from build123d import *

# Parameters (mm, degrees)
PAD_DEPTH          = 11
SKETCH001_R        = 2
PAD001_DEPTH       = 0.4
SKETCH002_R        = 0.5
PAD002_DEPTH       = 3.8
SKETCH003_R        = 0.5
POCKET_DEPTH       = 3
SKETCH004_R        = 2.5
SKETCH004_R_2      = 1
PAD003_DEPTH       = 1.2
SKETCH005_W        = 3
SKETCH005_H        = 1.8
POCKET001_DEPTH    = 2
SKETCH006_W        = 0.3
SKETCH006_H        = 1.478048
PAD004_DEPTH       = 2
POCKET002_DEPTH    = 0.2
POLARPATTERN_COUNT = 2


with BuildPart() as part:
    # Sketch → Pad (new body, symmetric)
    with BuildSketch(Plane.XY):
        with BuildLine():
            ThreePointArc((-3.316625, 5), (-6, 0), (-3.316625, -5))
            Line((-3.316625, -5), (3.316625, -5))
            ThreePointArc((3.316625, -5), (6, 0), (3.316625, 5))
            Line((-3.316625, 5), (3.316625, 5))
        make_face()
    extrude(amount=PAD_DEPTH, both=True)

    # Sketch001 (on Face6 of Pad) → Pad001 (join)
    with BuildSketch(Plane.XY.offset(11)):
        Circle(SKETCH001_R)
    extrude(amount=PAD001_DEPTH)

    # Sketch002 (on Face8 of Pad001) → Pad002 (join)
    with BuildSketch(Plane.XY.offset(11.4)):
        Circle(SKETCH002_R)
    extrude(amount=PAD002_DEPTH)

    # Sketch003 (on Face5 of Pad002) → Pocket (cut)
    with BuildSketch(Plane.XY.offset(11)):
        with Locations((0, 3.6)):
            Circle(SKETCH003_R)
        with Locations((-4.3, 0)):
            Circle(SKETCH003_R)
        with Locations((4.3, 0)):
            Circle(SKETCH003_R)
    extrude(amount=-POCKET_DEPTH, mode=Mode.SUBTRACT)

    # Sketch004 (on Face4 of Pocket) → Pad003 (join)
    with BuildSketch(Plane(origin=(0, 0, -11), x_dir=(1, 0, 0), z_dir=(0, 0, -1))):
        Circle(SKETCH004_R)
        Circle(SKETCH004_R_2, mode=Mode.SUBTRACT)
    extrude(amount=PAD003_DEPTH)

    # Sketch005 (on Face4 of Pad003) → Pocket001 (cut)
    with BuildSketch(Plane(origin=(0, 0, -11), x_dir=(1, 0, 0), z_dir=(0, 0, -1))):
        with Locations((-6, 0)):
            Rectangle(SKETCH005_W, SKETCH005_H)
        with Locations((6, 0)):
            Rectangle(SKETCH005_W, SKETCH005_H)
    extrude(amount=-POCKET001_DEPTH, mode=Mode.SUBTRACT)

    # Sketch006 (on Face2 of Pocket001) → Pad004 (join)
    with BuildSketch(Plane(origin=(0, 0, -11), x_dir=(1, 0, 0), z_dir=(0, 0, -1))):
        with Locations((-3.95, 0)):
            Rectangle(SKETCH006_W, SKETCH006_H)
        with Locations((3.95, 0)):
            Rectangle(SKETCH006_W, SKETCH006_H)
    extrude(amount=PAD004_DEPTH)

    # Sketch007 (on Face6 of Pad004) → Pocket002 (cut)
    with BuildSketch(Plane.XZ.offset(5)):
        with BuildLine():
            ThreePointArc((-2.15, 2.4), (-2.4, 2.65), (-2.65, 2.4))
            Line((-2.65, 2.4), (-2.65, -2.4))
            ThreePointArc((-2.65, -2.4), (-2.4, -2.65), (-2.15, -2.4))
            Line((-2.15, 2.4), (-2.15, -2.4))
        make_face()
        with BuildLine():
            ThreePointArc((2.65, 2.4), (2.4, 2.65), (2.15, 2.4))
            Line((2.15, 2.4), (2.15, -2.4))
            ThreePointArc((2.15, -2.4), (2.4, -2.65), (2.65, -2.4))
            Line((2.65, 2.4), (2.65, -2.4))
        make_face()
    pocket002 = extrude(amount=-POCKET002_DEPTH, mode=Mode.SUBTRACT)

    # PolarPattern: Pocket002 ×2 about axis
    polarpattern_axis = Axis((0, 0, 0), (0, 0, 1))
    for i in range(1, POLARPATTERN_COUNT):
        add(pocket002.rotate(polarpattern_axis, i * 360 / POLARPATTERN_COUNT), mode=Mode.SUBTRACT)


solid = part.part
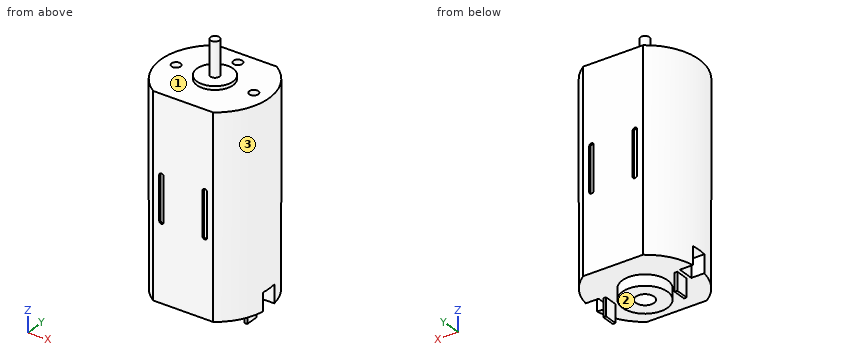
Verification items for the finished model (mm, model axes). Face numbers are marked on the shaded views. Coordinates: 2 decimals unless noted, no trailing zeros. Order: outer loops, then holes, each group sorted by start corner. A loop starts at its lowest first (then second) coordinate and runs counter-clockwise, first axis right, second up.
1. Scan lines: line 1 (X direction, y = 0, z = -11.65); line 2 (Y direction, x = 0, z = 9.6); line 3 (Y direction, x = 0, z = -11.5). Record each from-to range of solid material in increasing order.
Results found:
line 1: x = -4.1 to -3.8, -2.5 to -1, 1 to 2.5, 3.8 to 4.1
line 2: y = -5 to 3.1, 4.1 to 5
line 3: y = -2.5 to -1, 1 to 2.5
2. Sectioned sample at A-A, the plane z = -1. Record the cut outline in (x, y), and give its area (3 significant figures).
Results found:
outline: (-3.32, -5) - (-2.65, -5) - (-2.65, -4.8) - (-2.15, -4.8) - (-2.15, -5) - (2.15, -5) - (2.15, -4.8) - (2.65, -4.8) - (2.65, -5) - (3.32, -5) arc R6 ccw to (3.32, 5) - (2.65, 5) - (2.65, 4.8) - (2.15, 4.8) - (2.15, 5) - (-2.15, 5) - (-2.15, 4.8) - (-2.65, 4.8) - (-2.65, 5) - (-3.32, 5) arc R6 ccw to start
area: 104 mm2
3. Sectioned sample at D-D, the plane z = 12. Record the cut outline in (x, y), and give its area (3 significant figures).
Results found:
outline: circle Ø1 at (0, 0)
area: 0.785 mm2
4. Sectioned sample at C-C, the plane x = -1.5. Record the cut outline in (y, z), and give its area (3 significant figures).
Results found:
outline: (-5, -11) - (-2, -11) - (-2, -12.2) - (2, -12.2) - (2, -11) - (5, -11) - (5, 11) - (1.32, 11) - (1.32, 11.4) - (-1.32, 11.4) - (-1.32, 11) - (-5, 11) - close
area: 226 mm2
5. Release check for a two-part mould opening along X. For the marked faces 1, 2 and 3 record: +X half, -X half, draft (parallel to the pull), parting line (faces both ways), or undercut.
Results found:
face 1: draft
face 2: undercut
face 3: +X half
6. Sectioned sample at B-B, the plane y = 3.6. Record the cut outline in (x, z).
Results found:
outline: (-4.8, -11) - (4.8, -11) - (4.8, 11) - (0.5, 11) - (0.5, 8) - (-0.5, 8) - (-0.5, 11) - (-4.8, 11) - close
7. Go/stop test with flat-tipped pins: pin 1 Ø0.7 at (x, z) = (5, -10) entering from -Y; pin 2 Ø1 at (x, z) = (4.5, 2) entering from -Y; pin 3 Ø2 at (y, z) = (4, 1.5) entering from +X. Record where each tip stops, or that it passes through.
Results found:
pin 1: stops at y = -3.79
pin 2: stops at y = -4.47
pin 3: stops at x = 5.2
